Input: dimensioned drawing with shaded views. Units: mm. Origin: part minimum x, y, z. A direction names the side the tool comes from. Coordinates: 2 decimals unless noted, no trailing zeros. Loops run counter-clockwise (first coordinate to the right, second up) from the corner with the lowest first, then second, coordinate; pieces in that order, holes last.
Item 1: Section A-A on y = 14.75. Return loops of the section in (x, z).
Item 2: Reachability of the marked faces 1 and 2 from +Z, -Z, +X, -X, +Y, -Y: full face, straight path, thin tool, end or side. Return the list, or none.
Item 3: Contact query for flat-ended pins moving along their axis: P1, Ø4, axis at y = 6, z = 25, coming from the +X side; P2, Ø4, axis at y = 10, z = 23.5, coming from the -X side; P3, Ø1.5, axis at x = 10.5, z = 12.5, coming from the -Y side; P4, Ø11.5, axis at x = 16.5, z = 15, coming from the -Y side. Output: stop coordinate, or through.
Item 4: Ray query, line 1 along Z through (x, y) = (16.8, 4.9) (3 decimals); line 2 along X through (y, z) = (17.5, 16.8) (3 decimals). Return the intervals inside material, ascending.
Item 5: Pull-direction query (X, two-part tool) for the marked faces 3, 4 and 5; classes: released by +X, released by -X, zero draft, split by the parting line, or undercut.
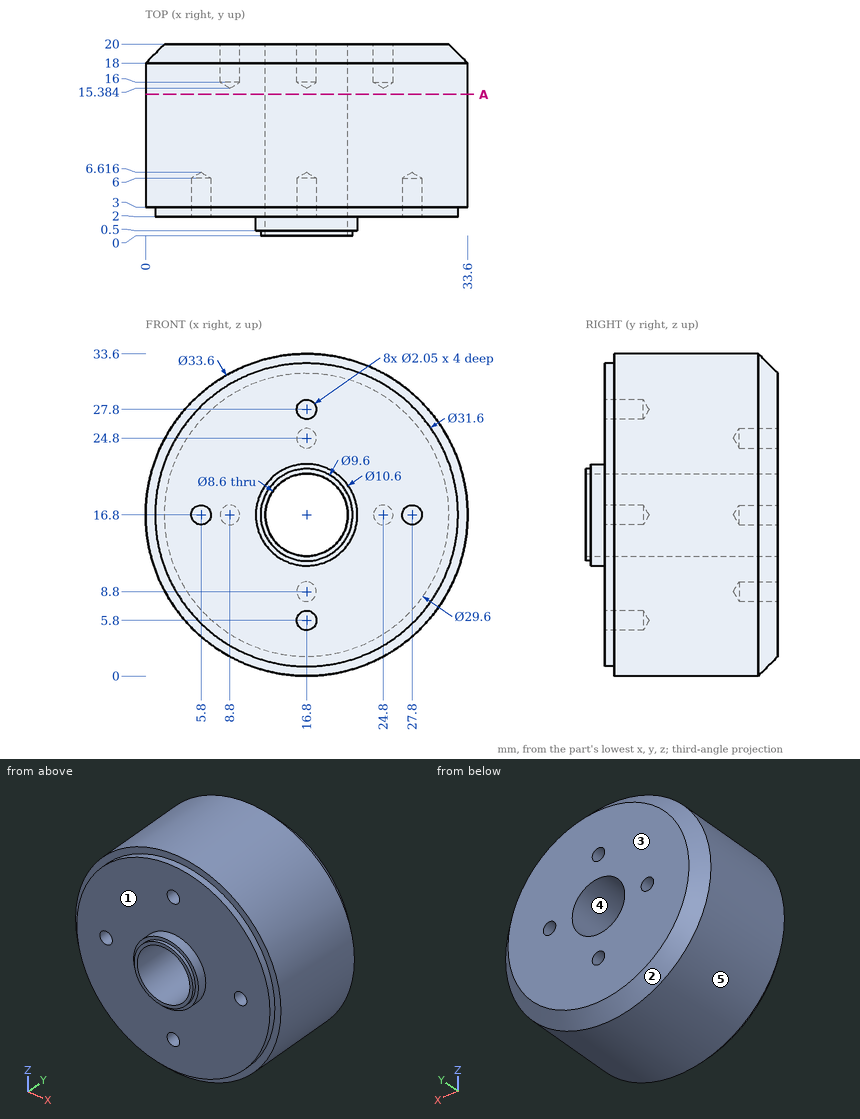
Results found:
1. outline: circle Ø33.6 at (16.8, 16.8); hole circle Ø8.6 at (16.8, 16.8)
2. face 1: -Y
2. face 2: +Y
3. P1: stops at x = 32.41
3. P2: stops at x = 0.67
3. P3: stops at y = 2
3. P4: stops at y = 0
4. line 1: z = 0 to 4.775, 6.825 to 12.5, 21.1 to 26.775, 28.825 to 33.6
4. line 2: x = 0 to 7.775, 9.825 to 12.5, 21.1 to 23.775, 25.825 to 33.6
5. face 3: zero draft
5. face 4: undercut
5. face 5: split by the parting line
